The listing builds one solid part. Answer for the finished solid, in the listing's coordinates (mm). A direction names the side the tool comes from. Round coordinates to 2 decimals unless told otherwise and drop trailing zeros. Write each loop counter-clockwise with the first axis right and the second up, starting at its lowest first coordinate (ties: lowest second). Pieces come first, ordered by that corner, then holes. Notation, with made-up numbers: (19, 76) - (63, 76) arc R10 cw to (63, 95) - close; hole circle Ø7 at (52, 74). An arc over 180 degrees is marked (long way). Use a Markdown table: item, result. Add a question column.
1) A cutting plane is placed at A-A (z = 58). Give the vertices of the cut face in (x, y), then the cut area to 3 significant figures.
2) Determine the mould class of faces 3 (the flat face through (56.324, 0.496, 62.74)), 4 (the conical face through (21.42, 6.75, 47.76)), 5 (the cylindrical face through (-56.007, -42.438, 30.524)) for opening direction Y: +Y half, -Y half, draft (parallel to the pull), parting line (faces both ways), or undercut.
3) Find the intervals of material crossed by probe 1 along Y at (x, z) = (0, 56); probe 2 along Z at (x, y) = (-0.5, 12.5); probe 3 along X at (y, z) = (-14.5, 60.5), in increasing order. Write a range as from..to.
4) A tool of negligible diameter and unlimited length cuts with its end or side. For faces 1 (the cylindrical face through (-5.9, -26.568, 56.414)), 2 (the flat face through (-37, 1, 65.205)), from which of +Z, -Z, +X, -X, +Y, -Y can it reach the whole face along a straight path? Write none if from no direction.
5) A cutting plane is placed at B-B (x = 0). Give the vertices of the cut face in (y, z), then the cut area to 3 significant figures.
6) A cutting plane is placed at C-C (y = 0). Give the vertices of the cut face in (x, z), then the cut area to 3 significant figures.
7) Each of these flat-tipped pins is pushed along its axis until it touches: P1, Ø13.5, axis at x = -3.5, y = -8.5, coming from the +Z side; P2, Ø8, axis at x = 43, y = -24.5, coming from the -Z side; P3, Ø2, axis at x = 4, y = 28.5, coming from the +Z side. Where does it stop, or does it pass through?
```python
from build123d import *

# Parameters (mm, degrees)
F0_W     = 117.717252
F0_H     = 90.889574
F1_DEPTH = 65.204948
F2_R     = 10
F3_SIZE  = 5
F4_R     = 27.215053
F5_DEPTH = 17.689077
F6_SIZE  = 5


with BuildPart() as f1:
    # F0 (on Top) → F1 (new body)
    with BuildSketch(Plane.XY):
        Rectangle(F0_W, F0_H)
    extrude(amount=F1_DEPTH)

    # F2
    f2_edges = [f1.edges().sort_by_distance(p)[0] for p in [
        (-58.858626, 45.444787, 32.602474),
        (-58.858626, -45.444787, 32.602474),
        (58.858626, -45.444787, 32.602474),
        (58.858626, 45.444787, 32.602474),
    ]]
    fillet(f2_edges, radius=F2_R)

    # F3
    f3_edges = [f1.edges().sort_by_distance(p)[0] for p in [
        (-58.858626, 0, 65.204948),
        (-55.929693, 42.515854, 65.204948),
        (-55.929693, -42.515854, 65.204948),
        (0, 45.444787, 65.204948),
        (0, -45.444787, 65.204948),
        (55.929693, 42.515854, 65.204948),
        (55.929693, -42.515854, 65.204948),
        (58.858626, 0, 65.204948),
    ]]
    chamfer(f3_edges, length=F3_SIZE)

    # F4 (on face) → F5 (cut)
    with BuildSketch(Plane.XY.offset(65.204948)):
        Circle(F4_R)
    extrude(amount=-F5_DEPTH, mode=Mode.SUBTRACT)

    # F6
    f6_edges = [f1.edges().sort_by_distance(p)[0] for p in [
        (27.215053, 0, 56.36041),
        (-27.215053, 0, 65.204948),
        (-27.215053, 0, 47.515871),
    ]]
    chamfer(f6_edges, length=F6_SIZE)


solid = f1.part
```
Entries:
| question | item | result |
|---|---|---|
| 1 | outline | (-58.86, -35.44) arc R10 ccw to (-48.86, -45.44) - (48.86, -45.44) arc R10 ccw to (58.86, -35.44) - (58.86, 35.44) arc R10 ccw to (48.86, 45.44) - (-48.86, 45.44) arc R10 ccw to (-58.86, 35.44) - close; hole circle Ø54.43 at (0, 0) |
| 1 | area | 8,290 mm² |
| 2 | face 3 | draft |
| 2 | face 4 | undercut |
| 2 | face 5 | -Y half |
| 3 | probe 1 | y = -45.44..-27.22, 27.22..45.44 |
| 3 | probe 2 | z = 0..47.52 |
| 3 | probe 3 | x = -58.56..-23.38, 23.38..58.56 |
| 4 | face 1 | +Z |
| 4 | face 2 | +Z, +X, -X, +Y, -Y |
| 5 | outline | (-45.44, 0) - (45.44, 0) - (45.44, 60.2) - (40.44, 65.2) - (32.22, 65.2) - (27.22, 60.2) - (27.22, 52.52) - (22.22, 47.52) - (-22.22, 47.52) - (-27.22, 52.52) - (-27.22, 60.2) - (-32.22, 65.2) - (-40.44, 65.2) - (-45.44, 60.2) - close |
| 5 | area | 4,940 mm² |
| 6 | outline | (-58.86, 0) - (58.86, 0) - (58.86, 60.2) - (53.86, 65.2) - (32.22, 65.2) - (27.22, 60.2) - (27.22, 52.52) - (22.22, 47.52) - (-22.22, 47.52) - (-27.22, 52.52) - (-27.22, 60.2) - (-32.22, 65.2) - (-53.86, 65.2) - (-58.86, 60.2) - close |
| 6 | area | 6,690 mm² |
| 7 | P1 | stops at z = 47.52 |
| 7 | P2 | stops at z = 0 |
| 7 | P3 | stops at z = 62.77 |
